Autodesk Inventor part; units mm, degrees
ref_plane "YZ Plane" through (0, 0, 0) normal (1, 0, 0) x (0, 1, 0)
ref_plane "XZ Plane" through (0, 0, 0) normal (0, 1, 0) x (-1, 0, 0)
ref_plane "XY Plane" through (0, 0, 0) normal (0, 0, 1) x (1, 0, 0)
sketch "Эскиз1" plane through (0, 0, 0) normal (0, 1, 0) x (-1, 0, 0)
  line L0 (42, 40) -> (42, 38)
  line L1 (-28.1339, -42) -> (-42.25, -42)
  line L2 (42, 40) -> (-42.25, 40)
  line L3 (-42.25, 40) -> (-42.25, -42)
  line L4 (-42.25, -42) -> (42, -42)
  line L5 (42, -42) -> (42, 40)
  circle A0 centre (39.5, -17) radius 1.5
  circle A1 centre (-39.75, -17) radius 1.5
  circle A2 centre (-39.75, 17) radius 1.5
  circle A3 centre (39.5, 17) radius 1.5
  point P0 (0, 0)
  point P1 (0, 0)
extrude "Выдавливание1" add sketch "Эскиз1" along normal blind 4
fillet "Сопряжение1" radius 10 4 edges at (42.25, 2, 40) (42.25, 2, -42) (-42, 2, -42) (-42, 2, 40)
properties part number "KB33-046-004-021 - Зажим точки доступа"
Here's how the part is built. I have some questions about the finished solid (model axes, mm). Give positions to 0.01 mm unless a question says otherwise; leave off trailing zeros. Order: outer loops, then holes, each group sorted by start corner. A loop starts at its lowest first (then second) coordinate and runs counter-clockwise, first axis right, second up. Notation, with made-up numbers: (-16.5, 41.5) - (13.5, 41.5) arc R31 ccw to (13.5, 67.5) - close; hole circle Ø10 at (54.5, -0.5). An arc over 180 degrees is marked (long way). Answer as a JSON object with one key per item and string values. Group by question number.
Item 1: Please list where these lines run through material, in increasing order: probe 1 along Z at (x, y) = (-39.5, 3.1); probe 2 along Z at (x, y) = (35.5, 3.8); probe 3 along X at (y, z) = (2.2, -35.5).
Item 2: If we section it at A-A on z = -17: Please give me the cut outline in (x, y), and give its area (3 significant figures).
Item 3: If we section it at C-C on y = 2.7: Give the number of separate pieces and of enclosed holes in the cut face, and give its area (3 significant figures).
Item 4: For P1, Ø2.5, axis at x = 39.75, z = -17, coming from the -Y side, with a flat end and sliding along its axis, tell me the tip position at first contact or that it passes through.
Item 5: If we mould it in two halves opening along Z, with no side actions, what happens to faces 1 (the flat face through (0, 2, -42)), 2 (the flat face through (0, 2, 40)), 3 (the cylindrical face through (-38.39, 1.97, -18.01))? For each: pulls with the +Z half, pulls with the -Z half, needs draft (parallel to the pull), parting line crosses it, or undercut.
Item 6: If we section it at B-B on x = 39.75: Please give me the cut outline in (y, z), and give its area (3 significant figures).
Result set:
{
 "1": {"probe 1": "-38.61 to -18.5, -15.5 to 15.5, 18.5 to 36.61", "probe 2": "-41.46 to 39.46", "probe 3": "-41.37 to 41.62"},
 "2": {"outline": "(-42, 0) - (-41, 0) - (-41, 4) - (-42, 4) - close; (-38, 0) - (38.25, 0) - (38.25, 4) - (-38, 4) - close; (41.25, 0) - (42.25, 0) - (42.25, 4) - (41.25, 4) - close", "area": "313 mm²"},
 "3": {"separate pieces": "1", "enclosed holes": "4", "area": "6,790 mm²"},
 "4": {"P1": "through"},
 "5": {"face 1": "pulls with the -Z half", "face 2": "pulls with the +Z half", "face 3": "undercut"},
 "6": {"outline": "(0, -38.61) - (4, -38.61) - (4, -18.5) - (0, -18.5) - close; (0, -15.5) - (4, -15.5) - (4, 15.5) - (0, 15.5) - close; (0, 18.5) - (4, 18.5) - (4, 36.61) - (0, 36.61) - close", "area": "277 mm²"}
}
